```python
from build123d import *

# Parameters (mm, degrees)
SKETCH_R  = 2.55
PAD_DEPTH = 58
FILLET_R  = 1


with BuildPart() as part:
    # Sketch → Pad (new body)
    with BuildSketch(Plane.XY):
        Polygon((-5, 0), (-2.5, -4.330127), (2.5, -4.330127), (5, 0), (2.5, 4.330127), (-2.5, 4.330127), align=None)
        Circle(SKETCH_R, mode=Mode.SUBTRACT)
    extrude(amount=PAD_DEPTH)

    # Fillet
    fillet_edges = [part.edges().sort_by_distance(p)[0] for p in [
        (-2.55, 0, 0),
    ]]
    fillet(fillet_edges, radius=FILLET_R)


solid = part.part
```
Geometry check sheet. Reference: the model listing, model coordinates, mm. Round coordinates to 2 decimals unless told otherwise and drop trailing zeros. Order: outer loops, then holes, each group sorted by start corner. A loop starts at its lowest first (then second) coordinate and runs counter-clockwise, first axis right, second up. Notation, with made-up numbers: (67, 13) -> (75, 13) arc R12 cw to (75, 25) -> close; hole circle Ø2 at (-16.5, 63.5). An arc over 180 degrees is marked (long way). Return JSON: item names as keys, results as strings. Group by question number.
Q1. Release check for a two-part mould opening along X. For faces 1 (the flat face through (3.73, -2.2, 28.59)), 2 (the flat face through (-3.73, 2.2, 28.59)), 3 (the flat face through (0, -4.33, 29)), 4 (the cylindrical face through (1.18, -2.26, 29.1)) record: released by +X, released by -X, zero draft, split by the parting line, or undercut.
Q2. Section check A-A, the plane x = 0. Record the boundary of the cut face in (y, z).
Q3. Material ranges on probe 1 along Y at (x, z) = (0, 27.5); probe 2 along X at (y, z) = (0.75, 44); probe 3 along X at (y, z) = (-2, 38.5), recorded low to high. Write a range as from..to.
Q4. Gauge pin test, flat end, axial feed: pin 1 (1 mm diameter, centred on y = 2, z = 35, fed in from -X). Record the tip position at first contact, or that the pin passes through.
Q5. Section check B-B, the plane z = 13.5. Record the boundary of the cut face in (x, y).
Numbers:
{
 "1": {"face 1": "released by +X", "face 2": "released by -X", "face 3": "zero draft", "face 4": "undercut"},
 "2": {"outline": "(-4.33, 0) -> (-3.55, 0) arc R1 ccw to (-2.55, 1) -> (-2.55, 58) -> (-4.33, 58) -> close; (2.55, 1) arc R1 ccw to (3.55, 0) -> (4.33, 0) -> (4.33, 58) -> (2.55, 58) -> close"},
 "3": {"probe 1": "-4.33..-2.55, 2.55..4.33", "probe 2": "-4.57..-2.44, 2.44..4.57", "probe 3": "-3.85..-1.58, 1.58..3.85"},
 "4": {"pin 1": "x = -4.13"},
 "5": {"outline": "(-5, 0) -> (-2.5, -4.33) -> (2.5, -4.33) -> (5, 0) -> (2.5, 4.33) -> (-2.5, 4.33) -> close; hole circle Ø5.1 at (0, 0)"}
}
